from build123d import *

# Parameters (mm, degrees)
SKETCH_1_W           = 104
SKETCH_1_H           = 64
EXTRUDE_1_DEPTH      = 3
SKETCH_2_R           = 1.5
CUT_EXTRUDE_1_DEPTH  = 62.131006862
SKETCH_4_R           = 2
CUT_EXTRUDE_3_DEPTH  = 1
SKETCH_12_W          = 5
SKETCH_12_H          = 12
EXTRUDE_4_DEPTH      = 0.5
SKETCH_13_R          = 0.5
CUT_EXTRUDE_8_DEPTH  = 62.15758334
SKETCH_15_W          = 22
SKETCH_15_H          = 12
CUT_EXTRUDE_10_DEPTH = 62.131006862
SKETCH_17_W          = 6.358168499
SKETCH_17_H          = 19.16029301
CUT_EXTRUDE_11_DEPTH = 4
FILLET_2_R           = 3
SKETCH_18_R          = 3
CUT_EXTRUDE_12_DEPTH = 6


with BuildPart() as part:
    # 草图1 → 凸台-拉伸1 (new body)
    with BuildSketch(Plane.XY):
        Rectangle(SKETCH_1_W, SKETCH_1_H)
    extrude(amount=EXTRUDE_1_DEPTH)

    # 草图2 → 切除-拉伸1 (cut, through all)
    with BuildSketch(Plane.XY.offset(3)):
        with Locations((-48, 28)):
            Circle(SKETCH_2_R)
        with Locations(Location((48, 28, 0), (0, 0, 180))):
            Circle(SKETCH_2_R)
        with Locations((48, -28)):
            Circle(SKETCH_2_R)
        with Locations(Location((-48, -28, 0), (0, 0, 180))):
            Circle(SKETCH_2_R)
    extrude(amount=-CUT_EXTRUDE_1_DEPTH, mode=Mode.SUBTRACT)

    # 草图4 → 切除-拉伸3 (cut)
    with BuildSketch(Plane.XY.offset(3)):
        with Locations((48, 28)):
            Circle(SKETCH_4_R)
        with Locations(Location((-48, 28, 0), (0, 0, 180))):
            Circle(SKETCH_4_R)
        with Locations((-48, -28)):
            Circle(SKETCH_4_R)
        with Locations(Location((48, -28, 0), (0, 0, 180))):
            Circle(SKETCH_4_R)
    extrude(amount=-CUT_EXTRUDE_3_DEPTH, mode=Mode.SUBTRACT)

    # 草图12 → 凸台-拉伸4 (add)
    with BuildSketch(Plane.XY.offset(3)):
        with Locations((17.5, 0)):
            Rectangle(SKETCH_12_W, SKETCH_12_H)
        with Locations((44.5, 0)):
            Rectangle(SKETCH_12_W, SKETCH_12_H)
    extrude(amount=EXTRUDE_4_DEPTH)

    # 草图13 → 切除-拉伸8 (cut, through all)
    with BuildSketch(Plane.XY.offset(3.5)):
        with Locations((17.5, 0)):
            Circle(SKETCH_13_R)
        with Locations((44.5, 0)):
            Circle(SKETCH_13_R)
    extrude(amount=-CUT_EXTRUDE_8_DEPTH, mode=Mode.SUBTRACT)

    # 草图15 → 切除-拉伸10 (cut, through all)
    with BuildSketch(Plane.XY.offset(3)):
        with Locations((31, 0)):
            Rectangle(SKETCH_15_W, SKETCH_15_H)
    extrude(amount=-CUT_EXTRUDE_10_DEPTH, mode=Mode.SUBTRACT)

    # 草图17 → 切除-拉伸11 (cut)
    with BuildSketch(Plane.XY.offset(3)):
        with Locations((38.820915751, 0)):
            Rectangle(SKETCH_17_W, SKETCH_17_H)
    extrude(amount=-CUT_EXTRUDE_11_DEPTH, mode=Mode.SUBTRACT)

    # 圆角2
    fillet_2_edges = [part.edges().sort_by_distance(p)[0] for p in [
        (35.641831501, -7.790073253, 3),
        (38.82091575, -9.580146505, 3),
        (42, -7.790073253, 3),
        (42, 7.790073253, 3),
        (38.82091575, 9.580146505, 3),
        (35.641831501, 7.790073253, 3),
    ]]
    fillet(fillet_2_edges, radius=FILLET_2_R - 0.0001)  # a hair under: the kernel refuses the full size

    # 草图18 → 切除-拉伸12 (cut)
    with BuildSketch(Plane.XY.offset(3)):
        with Locations((-42, -0.800014708)):
            Circle(SKETCH_18_R)
    extrude(amount=-CUT_EXTRUDE_12_DEPTH, mode=Mode.SUBTRACT)


solid = part.part
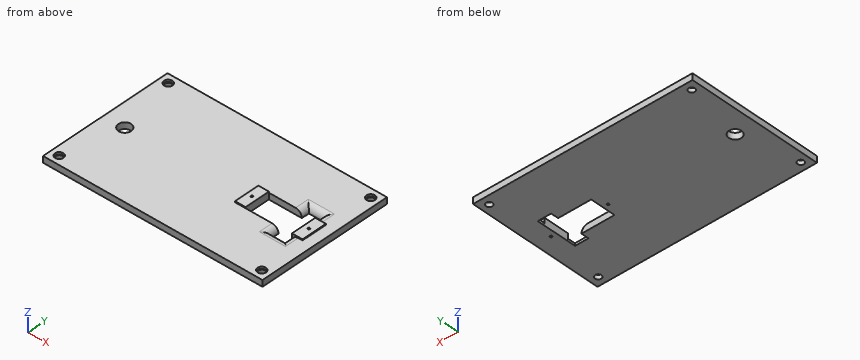
The model under review builds one solid part; all positions refer to its coordinate system, in mm. Coordinates: 2 decimals unless noted, no trailing zeros. Order: outer loops, then holes, each group sorted by start corner. A loop starts at its lowest first (then second) coordinate and runs counter-clockwise, first axis right, second up. Notation, with made-up numbers: (-19.75, 67.5) -> (-10.75, 67.5) arc R23 cw to (-10.75, 76.5) -> close; hole circle Ø8 at (47, 51). An arc over 180 degrees is marked (long way). Answer in a Markdown table with one row per item.
(1) Consider section B-B (y = 4.5). Write out the cut boundary in (x, z).
Answers:
| item | result |
|---|---|
| outline | (-52, 0) -> (20, 0) -> (20, 3.5) -> (15, 3.5) -> (15, 3) -> (-52, 3) -> close; (42, 0) -> (52, 0) -> (52, 3) -> (47, 3) -> (47, 3.5) -> (42, 3.5) -> close |
(2) Consider section A-A (x = -48). Write out the cut boundary in (y, z).
Answers:
| item | result |
|---|---|
| outline | (-32, 0) -> (-29.5, 0) -> (-29.5, 2) -> (-30, 2) -> (-30, 3) -> (-32, 3) -> close; (-26.5, 0) -> (26.5, 0) -> (26.5, 2) -> (26, 2) -> (26, 3) -> (-26, 3) -> (-26, 2) -> (-26.5, 2) -> close; (29.5, 0) -> (32, 0) -> (32, 3) -> (30, 3) -> (30, 2) -> (29.5, 2) -> close |
(3) Consider section D-D (z = 1.2). State how many separate pieces and enclosed holes the cut face has, plus the area to 3 significant figures.
Answers:
| item | result |
|---|---|
| separate pieces | 1 |
| enclosed holes | 8 |
| area | 6,280 mm² |
(4) Wall thickness on line 1 along Y through (x, z) = (-48, 1.3); line 2 along Y through (x, z) = (48, 2.85); line 3 along X through (y, z) = (9.5, 0.35): over which ranges is each line inside the solid? List them lowest first.
Answers:
| item | result |
|---|---|
| line 1 | -32 to -29.5, -26.5 to 26.5, 29.5 to 32 |
| line 2 | -32 to -30, -26 to 26, 30 to 32 |
| line 3 | -52 to 35.62, 42.02 to 52 |
(5) Consider section C-C (y = -28). Write out the cut boundary in (x, z), plus the area to 3 significant figures.
Answers:
| item | result |
|---|---|
| outline | (-52, 0) -> (-49.5, 0) -> (-49.5, 2) -> (-50, 2) -> (-50, 3) -> (-52, 3) -> close; (-46.5, 0) -> (46.5, 0) -> (46.5, 2) -> (46, 2) -> (46, 3) -> (-46, 3) -> (-46, 2) -> (-46.5, 2) -> close; (49.5, 0) -> (52, 0) -> (52, 3) -> (50, 3) -> (50, 2) -> (49.5, 2) -> close |
| area | 292 mm² |
(6) Insertion check: pin 1 (3 mm diameter, centred on x = 47.5, y = -27, fed in from +Z). The pin has a flat end and moves straight along its axis. Give the tip position at first contact, or say it passes through.
Answers:
| item | result |
|---|---|
| pin 1 | z = 3 |
